```python
from build123d import *

# Parameters (mm, degrees)
CYLINDER002_R                 = 2
CYLINDER002_DEPTH             = 30
CYLINDER002_PITCH_ANGLE       = 90
ROTATEEXTRUDE_ROLL_ANGLE      = 90
CYLINDER001_R                 = 20
CYLINDER001_DEPTH             = 9
CUBE_W                        = 3
CUBE_H                        = 5
CUBE_DEPTH                    = 16
CYLINDER_R                    = 8
CYLINDER_DEPTH                = 16
DIFFERENCE002_ROLL_ANGLE      = 180
DIFFERENCE002_PLACEMENT_ANGLE = 90


with BuildPart() as cylinder002:
    # cylinder002 → cylinder002 (new body)
    with BuildSketch(Plane.XY):
        Circle(CYLINDER002_R)
    extrude(amount=CYLINDER002_DEPTH)


with BuildPart() as cylinder002_1:
    # cylinder002 pitch: moved
    add(cylinder002.part.rotate(Axis((0, 0, 0), (0, 1, 0)), CYLINDER002_PITCH_ANGLE))


with BuildPart() as cylinder002_2:
    # cylinder002 placement: moved
    add(cylinder002_1.part.moved(Location((-15, 0, 12.5))))


with BuildPart() as rotateextrude:
    # RefineRotateExtrude → RotateExtrude (revolve)
    with BuildSketch(Plane(origin=(21.25, 4.242641, 0), x_dir=(0, 1, 0), z_dir=(0, 0, 1))):
        Polygon((0, 4.242641), (-4.242641, 0), (0, -4.242641), (4.242641, 0), align=None)
    revolve(axis=Axis((0, 0, 0), (0, 1, 0)))


with BuildPart() as rotateextrude_1:
    # RotateExtrude roll: moved
    add(rotateextrude.part.rotate(Axis((0, 0, 0), (1, 0, 0)), ROTATEEXTRUDE_ROLL_ANGLE))


with BuildPart() as rotateextrude_2:
    # RotateExtrude placement: moved
    add(rotateextrude_1.part)


with BuildPart() as cylinder001:
    # cylinder001 → cylinder001 (new body)
    with BuildSketch(Plane.XY):
        Circle(CYLINDER001_R)
    extrude(amount=CYLINDER001_DEPTH)


with BuildPart() as cube:
    # cube → cube (new body)
    with BuildSketch(Plane(origin=(-1.5, -2.5, 0), x_dir=(1, 0, 0), z_dir=(0, 0, 1))):
        with Locations((1.5, 2.5)):
            Rectangle(CUBE_W, CUBE_H)
    extrude(amount=CUBE_DEPTH)


with BuildPart() as obj1:
    # cylinder → cylinder (new body)
    with BuildSketch(Plane.XY):
        Circle(CYLINDER_R)
    extrude(amount=CYLINDER_DEPTH)

    # difference: cut cube
    add(cube.part, mode=Mode.SUBTRACT)

    # Group: union cylinder001
    add(cylinder001.part)

    # difference001: cut RotateExtrude
    add(rotateextrude_2.part, mode=Mode.SUBTRACT)

    # difference002: cut cylinder002
    add(cylinder002_2.part, mode=Mode.SUBTRACT)


with BuildPart() as obj1_1:
    # difference002 roll: moved
    add(obj1.part.rotate(Axis((0, 0, 0), (1, 0, 0)), DIFFERENCE002_ROLL_ANGLE))


with BuildPart() as obj1_2:
    # difference002 placement: moved
    add(obj1_1.part.moved(Location((0, 8, 35.6))).rotate(Axis((0, 8, 35.6), (0, 0, 1)), DIFFERENCE002_PLACEMENT_ANGLE))


solid = obj1_2.part
```
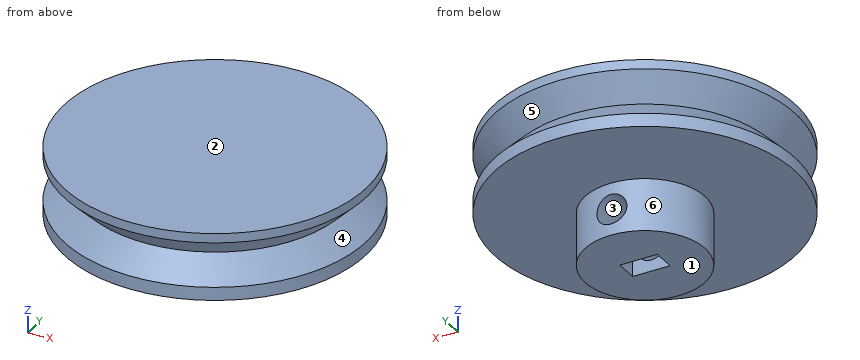
Read the model definition and answer for the solid it produces. Units are mm, in the model's axes. Face numbers are marked on the shaded views. A direction names the side the tool comes from. Round coordinates to 2 decimals unless told otherwise and drop trailing zeros. Write each loop counter-clockwise with the first axis right and the second up, starting at its lowest first coordinate (ties: lowest second). Pieces come first, ordered by that corner, then holes. Notation, with made-up numbers: (73, -14) - (94, -14) arc R13 cw to (94, 5) - close; hole circle Ø1 at (-28.5, -30.5). An arc over 180 degrees is marked (long way). Use CSV: the item, a comma, the result in double quotes.
Q1. Find section B-B, the plane x = 0. Write down the section's boundary in (y, z), then the cut area to 3 significant figures.
Values:
outline,"(-12, 26.6) - (0, 26.6) - (0, 25.1) - (6.5, 25.1) - (6.5, 26.6) - (9.5, 26.6) - (9.5, 25.1) - (16, 25.1) - (16, 26.6) - (28, 26.6) - (28, 28.36) - (25.01, 31.36) - (28, 34.35) - (28, 35.6) - (-12, 35.6) - (-12, 34.35) - (-9.01, 31.36) - (-12, 28.36) - close; (0, 19.6) - (6.5, 19.6) - (6.5, 21.1) - (0, 21.1) - close; (9.5, 19.6) - (16, 19.6) - (16, 21.1) - (9.5, 21.1) - close"
area,"381 mm²"
Q2. Find section D-D, the plane z = 30.75. Write down the section's boundary in (x, y).
Values:
outline,"circle Ø35.23 at (0, 8)"
Q3. Each of these flat-tipped pins is pushed along its axis until it touches: pin 1 Ø5 at (x, z) = (0, 23.1) entering from +Y; pin 2 Ø6 at (y, z) = (11, 31) entering from -X; pin 3 Ø8 at (y, z) = (14, 30.5) entering from +X; pin 4 Ø3 at (x, z) = (0, 23.1) entering from +Y. Where does it stop, or does it pass through?
Values:
pin 1,"stops at y = 16"
pin 2,"stops at x = -19.94"
pin 3,"stops at x = 19.83"
pin 4,"passes through"
Q4. Straight lines are drawn through the part: line 1 along Z through (x, y) = (14, 7); line 2 along X through (y, z) = (2, 22); line 3 along Z through (x, y) = (0.5, 4.5). For each, find the intervals that lie inside material, in ascending order.
Values:
line 1,"z = 26.6 to 35.6"
line 2,"x = -5.29 to -1.67, 1.67 to 5.29"
line 3,"z = 19.6 to 21.16, 25.04 to 35.6"
Q5. A tool of negligible diameter and unlimited length cuts with its end or side. For the marked faces 5 and 6, from which of +Z, -Z, +X, -X, +Y, -Y can it reach the whole face along a straight path? Write none if from no direction.
Values:
face 5,"none"
face 6,"-Z"
Q6. Find section C-C, the plane y = 8. Write down the section's boundary in (x, z), then the cut area to 3 significant figures.
Values:
outline,"(-20, 26.6) - (-8, 26.6) - (-8, 19.6) - (-2.5, 19.6) - (-2.5, 26.6) - (2.5, 26.6) - (2.5, 19.6) - (8, 19.6) - (8, 26.6) - (20, 26.6) - (20, 28.36) - (17.01, 31.36) - (20, 34.35) - (20, 35.6) - (-20, 35.6) - (-20, 34.35) - (-17.01, 31.36) - (-20, 28.36) - close"
area,"419 mm²"
Q7. Find section A-A, the plane z = 22. Write down the section's boundary in (x, y).
Values:
outline,"(-2.5, 6.5) - (-2.5, 9.5) - (-1.67, 9.5) - (-1.67, 15.82) arc R8 ccw to (-1.67, 0.18) - (-1.67, 6.5) - close; (1.67, 0.18) arc R8 ccw to (1.67, 15.82) - (1.67, 9.5) - (2.5, 9.5) - (2.5, 6.5) - (1.67, 6.5) - close"
Q8. Determine the mould class of the marked faces 1, 2, 3 and 4 for opening direction Z: +Z half, -Z half, draft (parallel to the pull), parting line (faces both ways), or undercut.
Values:
face 1,"-Z half"
face 2,"+Z half"
face 3,"undercut"
face 4,"undercut"
